Design review of the part built by this model. Coordinates are the model's own, in mm. A direction names the side the tool comes from. Round coordinates to 2 decimals unless told otherwise and drop trailing zeros. Write each loop counter-clockwise with the first axis right and the second up, starting at its lowest first coordinate (ties: lowest second). Pieces come first, ordered by that corner, then holes. Notation, with made-up numbers: M 70.25,5 L 101.25,5 A7 cw 101.25,11 Z; hole C -16.5,6 d6. An arc over 180 degrees is marked long. One line per question, with ' | ' between items. Start each with the question number.
Item 1: Machinability: for faces 5 (the face through (31.776, 1.014, -214.286)), 6 (the face through (73, 0, -61)), which of the approach directions +Z, -Z, +X, -X, +Y, -Y give a long, thin tool a straight path to every point of the face, cutting with its end or side? Answer none if there is none.
Item 2: Add section A-A, the plane z = -160.5. State the section outline as (x, y) points.
Item 3: Add section B-B, the plane x = -43.5. State the section outline as (y, z) points, and give its area (3 significant figures).
Item 4: Insertion check: pin 1 Ø1.8 at (x, z) = (-4.77, -12.31) entering from -Y; pin 2 Ø1 at (y, z) = (1, 13) entering from +X. Each pin has a flat end and moves straight along its axis. Give the tip position at first contact, or say it passes through.
Item 5: Add section D-D, the plane x = 103. State the section outline as (y, z) points, and give its area (3 significant figures).
Item 6: Add section C-C, the plane y = 1.6. Give the number of separate pieces and of enclosed holes in the cut face, and give its area (3 significant figures).
Item 7: For L1, parallel to Z at x = -39, y = 1.6; L2, parallel to X at y = 0.9, z = -202.5; L3, parallel to X at y = 0.9, z = -174, list the stretches that pass through material, from the lowest coordinate up.
Item 8: Draft analysis for pull direction Z (two halves, no side actions). For faces 1 (the face through (-24.356, 0.986, -193.802)), 2 (the face through (172.37, 0.99, -193.37)), 3 (the face through (116.297, 1.014, -214.452)), 4 (the face through (73, 2, -61)), state which applies: released by +Z, released by -Z, zero draft, split by the parting line, or undercut.
```python
from build123d import *

# Parameters (mm, degrees)
ESQUISSE1_R      = 1.5
ESQUISSE1_R_2    = 9.5
EXTRUSION1_DEPTH = 2
EXTRUSION3_DEPTH = 311.873244438
ESQUISSE4_R      = 1.5
ESQUISSE4_R_2    = 2
EXTRUSION4_DEPTH = 10
ESQUISSE5_R      = 1.5
ESQUISSE5_R_2    = 2
EXTRUSION5_DEPTH = 10
EXTRUSION6_DEPTH = 10
ESQUISSE7_R      = 1.5
EXTRUSION7_DEPTH = 10
ESQUISSE8_R      = 1.5
EXTRUSION8_DEPTH = 10


with BuildPart() as part:
    # Esquisse1 → Extrusion1 (new body)
    with BuildSketch(Plane(origin=(0, 0, 0), x_dir=(1, 0, 0), z_dir=(0, 1, 0))):
        Polygon((215.226575971, 224.311602694), (-64.773424029, 224.311602694), (-64.773424029, 19.311602694), (-37.773424029, 19.311602694), (-37.773424029, -20.688397306), (-64.773424029, -20.688397306), (-64.773424029, -45.688397306), (215.226575971, -45.688397306), (215.226575971, -20.688397306), (188.226575971, -20.688397306), (188.226575971, 19.311602694), (215.226575971, 19.311602694), align=None)
        with Locations(Location((27.226575971, 12.311602694, 0), (0, 0, 270))):
            Circle(ESQUISSE1_R, mode=Mode.SUBTRACT)
        with Locations(Location((27.226575971, -13.688397306, 0), (0, 0, 270))):
            Circle(ESQUISSE1_R, mode=Mode.SUBTRACT)
        with Locations(Location((123.226575971, -13.688397306, 0), (0, 0, 90))):
            Circle(ESQUISSE1_R, mode=Mode.SUBTRACT)
        with Locations(Location((-54.773424029, -35.688397306, 0), (0, 0, 270))):
            Circle(ESQUISSE1_R, mode=Mode.SUBTRACT)
        with Locations(Location((205.226575971, -35.688397306, 0), (0, 0, 90))):
            Circle(ESQUISSE1_R, mode=Mode.SUBTRACT)
        with Locations(Location((-28.773424029, 12.311602694, 0), (0, 0, 270))):
            Circle(ESQUISSE1_R, mode=Mode.SUBTRACT)
        with Locations(Location((-28.773424029, -13.688397306, 0), (0, 0, 270))):
            Circle(ESQUISSE1_R, mode=Mode.SUBTRACT)
        with Locations(Location((-4.773424029, 12.311602694, 0), (0, 0, 270))):
            Circle(ESQUISSE1_R, mode=Mode.SUBTRACT)
        with Locations(Location((-4.773424029, -13.688397306, 0), (0, 0, 270))):
            Circle(ESQUISSE1_R, mode=Mode.SUBTRACT)
        with Locations(Location((165.226575971, -35.688397306, 0), (0, 0, 90))):
            Circle(ESQUISSE1_R, mode=Mode.SUBTRACT)
        with Locations(Location((155.226575971, -13.688397306, 0), (0, 0, 90))):
            Circle(ESQUISSE1_R, mode=Mode.SUBTRACT)
        with Locations(Location((155.226575971, 12.311602694, 0), (0, 0, 90))):
            Circle(ESQUISSE1_R, mode=Mode.SUBTRACT)
        with Locations(Location((179.226575971, -13.688397306, 0), (0, 0, 90))):
            Circle(ESQUISSE1_R, mode=Mode.SUBTRACT)
        with Locations(Location((179.226575971, 12.311602694, 0), (0, 0, 90))):
            Circle(ESQUISSE1_R, mode=Mode.SUBTRACT)
        with Locations(Location((-24.773424029, 184.311602694, 0), (0, 0, 270))):
            Circle(ESQUISSE1_R_2, mode=Mode.SUBTRACT)
        with Locations(Location((-38.773424029, 198.311602694, 0), (0, 0, 270))):
            Circle(ESQUISSE1_R, mode=Mode.SUBTRACT)
        with Locations(Location((-10.773424029, 170.311602694, 0), (0, 0, 270))):
            Circle(ESQUISSE1_R, mode=Mode.SUBTRACT)
        with Locations(Location((-38.773424029, 170.311602694, 0), (0, 0, 270))):
            Circle(ESQUISSE1_R, mode=Mode.SUBTRACT)
        with Locations(Location((-10.773424029, 198.311602694, 0), (0, 0, 270))):
            Circle(ESQUISSE1_R, mode=Mode.SUBTRACT)
        with Locations(Location((161.226575971, 198.311602694, 0), (0, 0, 90))):
            Circle(ESQUISSE1_R, mode=Mode.SUBTRACT)
        with Locations(Location((189.226575971, 170.311602694, 0), (0, 0, 90))):
            Circle(ESQUISSE1_R, mode=Mode.SUBTRACT)
        with Locations(Location((161.226575971, 170.311602694, 0), (0, 0, 90))):
            Circle(ESQUISSE1_R, mode=Mode.SUBTRACT)
        with Locations(Location((189.226575971, 198.311602694, 0), (0, 0, 90))):
            Circle(ESQUISSE1_R, mode=Mode.SUBTRACT)
        with Locations(Location((175.226575971, 184.311602694, 0), (0, 0, 90))):
            Circle(ESQUISSE1_R_2, mode=Mode.SUBTRACT)
        with Locations(Location((-14.773424029, -35.688397306, 0), (0, 0, 270))):
            Circle(ESQUISSE1_R, mode=Mode.SUBTRACT)
        with Locations(Location((75.226575971, -35.688397306, 0), (0, 0, 270))):
            Circle(ESQUISSE1_R, mode=Mode.SUBTRACT)
        with Locations(Location((123.226575971, 12.311602694, 0), (0, 0, 90))):
            Circle(ESQUISSE1_R, mode=Mode.SUBTRACT)
    extrude(amount=EXTRUSION1_DEPTH)

    # Esquisse3 → Extrusion3 (cut, through all)
    with BuildSketch(Plane(origin=(0, 2, 0), x_dir=(-1, 0, 0), z_dir=(0, 1, 0))):
        with BuildLine():
            Line((-35.226575971, -224.311602694), (-35.226575971, -124.311602694))
            ThreePointArc((-35.226575971, -124.311602694), (-73.226575971, -86.311602694), (-111.226575971, -124.311602694))
            Line((-111.226575971, -124.311602694), (-111.226575971, -224.311602694))
            Line((-111.226575971, -224.311602694), (-35.226575971, -224.311602694))
        make_face()
    extrude(amount=-EXTRUSION3_DEPTH, mode=Mode.SUBTRACT)

    # Esquisse4 → Extrusion4 (cut)
    with BuildSketch(Plane.XZ):
        with Locations(Location((-54.773424029, -192.811602694, 0), (0, 0, 270))):
            Circle(ESQUISSE4_R)
        with Locations(Location((-54.773424029, -52.811602694, 0), (0, 0, 270))):
            Circle(ESQUISSE4_R)
        with Locations(Location((205.226575971, -52.811602694, 0), (0, 0, 90))):
            Circle(ESQUISSE4_R)
        with Locations(Location((205.226575971, -192.811602694, 0), (0, 0, 90))):
            Circle(ESQUISSE4_R)
        with Locations(Location((-34.773424029, -214.311602694, 0), (0, 0, 270))):
            Circle(ESQUISSE4_R)
        with Locations(Location((-4.273424029, -214.311602694, 0), (0, 0, 270))):
            Circle(ESQUISSE4_R)
        with Locations(Location((171.726575971, -214.311602694, 0), (0, 0, 270))):
            Circle(ESQUISSE4_R)
        with Locations(Location((185.226575971, -214.311602694, 0), (0, 0, 90))):
            Circle(ESQUISSE4_R)
        with Locations(Location((15.726575971, -214.311602694, 0), (0, 0, 270))):
            Circle(ESQUISSE4_R)
        with Locations(Location((158.726575971, -216.811602694, 0), (0, 0, 270))):
            Circle(ESQUISSE4_R)
        with Locations(Location((25.226575971, -192.311602694, 0), (0, 0, 270))):
            Circle(ESQUISSE4_R)
        with Locations(Location((25.226575971, -112.311602694, 0), (0, 0, 270))):
            Circle(ESQUISSE4_R)
        with Locations(Location((144.726575971, -216.811602694, 0), (0, 0, 270))):
            Circle(ESQUISSE4_R)
        with Locations(Location((125.226575971, -205.311602694, 0), (0, 0, 270))):
            Circle(ESQUISSE4_R_2)
        with Locations(Location((145.226575971, -176.811602694, 0), (0, 0, 270))):
            Circle(ESQUISSE4_R)
        with Locations(Location((145.226575971, -198.311602694, 0), (0, 0, 270))):
            Circle(ESQUISSE4_R)
        with Locations(Location((135.226575971, -173.811602694, 0), (0, 0, 270))):
            Circle(ESQUISSE4_R_2)
    extrude(amount=-EXTRUSION4_DEPTH, mode=Mode.SUBTRACT)

    # Esquisse5 → Extrusion5 (cut)
    with BuildSketch(Plane(origin=(0, 2, 0), x_dir=(-1, 0, 0), z_dir=(0, 1, 0))):
        with Locations(Location((-131.226575971, -69.311602694, 0), (0, 0, 90))):
            Circle(ESQUISSE5_R)
        with Locations(Location((-122.226575971, -75.636158015, 0), (0, 0, 90))):
            Circle(ESQUISSE5_R_2)
        with Locations(Location((-151.829207664, -93.914234387, 0), (0, 0, 90))):
            Circle(ESQUISSE5_R)
        with Locations(Location((-161.829207664, -124.311602694, 0), (0, 0, 90))):
            Circle(ESQUISSE5_R)
        with Locations(Location((-83.226575971, -24.311602694, 0), (0, 0, 90))):
            Circle(ESQUISSE5_R_2)
        with Locations(Location((-94.226575971, -24.311602694, 0), (0, 0, 90))):
            Circle(ESQUISSE5_R)
        with Locations(Location((-192.226575971, -114.311602694, 0), (0, 0, 90))):
            Circle(ESQUISSE5_R)
        with Locations(Location((-182.226575971, -83.914234387, 0), (0, 0, 90))):
            Circle(ESQUISSE5_R)
    extrude(amount=-EXTRUSION5_DEPTH, mode=Mode.SUBTRACT)

    # Esquisse6 → Extrusion6 (cut)
    with BuildSketch(Plane(origin=(0, 2, 0), x_dir=(-1, 0, 0), z_dir=(0, 1, 0))):
        Polygon((-28.226575971, -224.311602694), (-38.226575971, -224.311602694), (-35.226575971, -204.537882761), align=None)
        Polygon((-111.226575971, -224.311602694), (-121.226575971, -224.311602694), (-111.226575971, -204.311602694), align=None)
    extrude(amount=-EXTRUSION6_DEPTH, mode=Mode.SUBTRACT)

    # Esquisse7 → Extrusion7 (cut)
    with BuildSketch(Plane(origin=(0, 2, 0), x_dir=(-1, 0, 0), z_dir=(0, 1, 0))):
        with Locations(Location((-71.726575971, -79.311602694, 0), (0, 0, 90))):
            Circle(ESQUISSE7_R)
        with Locations(Location((-78.726575971, -79.311602694, 0), (0, 0, 90))):
            Circle(ESQUISSE7_R)
    extrude(amount=-EXTRUSION7_DEPTH, mode=Mode.SUBTRACT)

    # Esquisse8 → Extrusion8 (cut)
    with BuildSketch(Plane(origin=(0, 2, 0), x_dir=(-1, 0, 0), z_dir=(0, 1, 0))):
        with Locations(Location((19.273424029, -23.811602694, 0), (0, 0, 90))):
            Circle(ESQUISSE8_R)
        with Locations(Location((4.273424029, -38.811602694, 0), (0, 0, 90))):
            Circle(ESQUISSE8_R)
    extrude(amount=-EXTRUSION8_DEPTH, mode=Mode.SUBTRACT)


solid = part.part
```
Computed values:
1) face 5: -Z, +Y, -Y | face 6: +Z, -Z, +X, -X, -Y
2) outline: M -64.77,0 L 35.23,0 L 35.23,2 L -64.77,2 Z; M 111.23,0 L 215.23,0 L 215.23,2 L 111.23,2 Z
3) outline: M 0,-224.31 L 2,-224.31 L 2,-19.31 L 0,-19.31 Z; M 0,20.69 L 2,20.69 L 2,45.69 L 0,45.69 Z | area: 460 mm^2
4) pin 1: passes through | pin 2: stops at x = 188.23
5) outline: M 0,-100.7 L 2,-100.7 L 2,45.69 L 0,45.69 Z | area: 293 mm^2
6) separate pieces: 1 | enclosed holes: 56 | area: 62,400 mm^2
7) L1: z = -224.31 to -199.79, -196.83 to -171.79, -168.83 to -19.31, 20.69 to 45.69 | L2: x = -64.77 to 35.23, 111.23 to 215.23 | L3: x = -64.77 to 35.23, 111.23 to 133.24, 137.22 to 215.23
8) face 1: undercut | face 2: undercut | face 3: released by -Z | face 4: zero draft
